Source: CAD feature listing. Evaluate the final solid. Frame: model axes, mm. A direction names the side the tool comes from. Give positions to 0.01 mm unless a question says otherwise; leave off trailing zeros. Order: outer loops, then holes, each group sorted by start corner. A loop starts at its lowest first (then second) coordinate and runs counter-clockwise, first axis right, second up. Notation, with made-up numbers: (-31.5, -11.75) - (-0.5, -11.75) arc R12 ccw to (-0.5, 2.25) - close; hole circle Ø2 at (57, 28). An arc over 180 degrees is marked (long way). Use CSV: the item, a comma, the result in double quotes.
```python
from build123d import *

# Parameters (mm, degrees)
SKETCH3_R               = 15.875
BOSS_EXTRUDE1_DEPTH     = 63.5
BOSS_EXTRUDE2_START     = -12.7
SKETCH4_W               = 63.5
SKETCH4_H               = 63.5
SKETCH4_R               = 15.875
SKETCH4_R_2             = 6.35
BOSS_EXTRUDE2_DEPTH     = 76.2
CUT_EXTRUDE1_REACH      = 147.497
CUT_EXTRUDE1_END_RADIUS = 6.35
SKETCH5_R               = 6.35


with BuildPart() as part:
    # Sketch3 → Boss-Extrude1 (new body)
    with BuildSketch(Plane(origin=(0, 0, 0), x_dir=(1, 0, 0), z_dir=(0, 1, 0))):
        with Locations(Location((0, 0, 0), (0, 0, 270))):
            Circle(SKETCH3_R)
    extrude(amount=BOSS_EXTRUDE1_DEPTH)


with BuildPart() as body_2:
    # Sketch4 → Boss-Extrude2 (new body)
    # profile 1 of 2: a face of its own
    with BuildSketch(Plane(origin=(0, 63.5, 0), x_dir=(1, 0, 0), z_dir=(0, 1, 0)).offset(BOSS_EXTRUDE2_START)):
        Rectangle(SKETCH4_W, SKETCH4_H)
        with Locations(Location((0, 0, 0), (0, 0, 270))):
            Circle(SKETCH4_R, mode=Mode.SUBTRACT)
    # profile 2 of 2: a face of its own
    with BuildSketch(Plane(origin=(0, 63.5, 0), x_dir=(1, 0, 0), z_dir=(0, 1, 0)).offset(BOSS_EXTRUDE2_START)):
        with Locations(Location((0, 0, 0), (0, 0, 270))):
            Circle(SKETCH4_R)
        with Locations(Location((0, 0, 0), (0, 0, 90))):
            Circle(SKETCH4_R_2, mode=Mode.SUBTRACT)
    extrude(amount=BOSS_EXTRUDE2_DEPTH)

    # Cut-Extrude1: up to this cylinder (the profile starts outside it)
    cut_extrude1_end = Plane(origin=(0, 95.25, 0), z_dir=(0, -1, 0)) * Cylinder(CUT_EXTRUDE1_END_RADIUS, 308.694, mode=Mode.PRIVATE)
    # Sketch5 → Cut-Extrude1 (cut, up to the surface)
    with BuildSketch(Plane.XY.offset(31.75), mode=Mode.PRIVATE) as cut_extrude1_sk1:
        with Locations((0, 95.25)):
            Circle(SKETCH5_R)
    cut_extrude1_tool1 = extrude(cut_extrude1_sk1.sketch, amount=-CUT_EXTRUDE1_REACH, mode=Mode.PRIVATE) - cut_extrude1_end
    add(cut_extrude1_tool1.solids().sort_by_distance((0, 95.25, 31.75))[0], mode=Mode.SUBTRACT)


with BuildPart() as part_1:
    add(part.part)

    # Combine1: union body 2
    add(body_2.part)


solid = part_1.part
```
Item 1: Section B-B on x = 0. Return the cut outline in (y, z) (3 decimals).
Filled in:
outline,"(0, -15.875) - (50.8, -15.875) - (50.8, -31.75) - (127, -31.75) - (127, -6.35) - (63.5, -6.35) - (63.5, 6.35) - (88.9, 6.35) - (88.9, 31.75) - (50.8, 31.75) - (50.8, 15.875) - (0, 15.875) - close; (101.6, 6.35) - (127, 6.35) - (127, 31.75) - (101.6, 31.75) - close"
Item 2: Mould query, pull axis X, two halves, no side actions, for faces 5 (the cylindrical face through (-1.907, 94.806, -6.057)), 6 (the flat face through (8, 127, 0)), 7 (the flat face through (-31.75, 88, 0)). Classes: released by +X, released by -X, zero draft, split by the parting line, or undercut.
Filled in:
face 5,"undercut"
face 6,"zero draft"
face 7,"released by -X"
Item 3: First-contact query: pin 1 (6 mm diameter, centred on x = 7.5, z = 19, fed in from -Y); pin 2 (1 mm diameter, centred on x = 4.5, y = 24.5, fed in from -Z); pin 3 (12 mm diameter, centred on x = -10.5, y = 22.5, fed in from +Z). Flat tips, straight axial feed; report the tip coordinate or a pass-through.
Filled in:
pin 1,"stops at y = 50.8"
pin 2,"stops at z = -15.36"
pin 3,"stops at z = 15.22"
Item 4: Section D-D on y = 95.25. Return the cut outline in (x, z).
Filled in:
outline,"(-31.75, -31.75) - (31.75, -31.75) - (31.75, 31.75) - (6.35, 31.75) - (6.35, 0) arc R6.35 cw to (-6.35, 0) - (-6.35, 31.75) - (-31.75, 31.75) - close"
Item 5: Section C-C on y = 74. Return the cut outline in (x, z).
Filled in:
outline,"(-31.75, -31.75) - (31.75, -31.75) - (31.75, 31.75) - (-31.75, 31.75) - close; hole circle Ø12.7 at (0, 0)"
Item 6: Set-up query: faces 1 (the cylindrical face through (-0.827, 101.546, 19.625)), 2 (the cylindrical face through (-15.497, 25.044, -3.441)), 3 (the flat face through (0, 88, 31.75)), 4 (the flat face through (0, 63.5, 0)). Return all of +Z, -Z, +X, -X, +Y, -Y with unobstructed straight access to the full face (end or side cutting, diameter ignored); none if empty.
Filled in:
face 1,"+Z"
face 2,"-Y"
face 3,"+Z, +X, -X, +Y, -Y"
face 4,"+Y"
Item 7: Section A-A on z = 20. Return the cut outline in (x, y).
Filled in:
outline,"(-31.75, 50.8) - (31.75, 50.8) - (31.75, 127) - (-31.75, 127) - close; hole circle Ø12.7 at (0, 95.25)"
Item 8: Material intervals for line 1 (X direction, y = 95.25, z = 9.5); line 2 (Y direction, x = 0, z = 13); line 3 (Y direction, x = -18, z = -18), sorted ascending. Write a range as from..to.
Filled in:
line 1,"x = -31.75..-6.35, 6.35..31.75"
line 2,"y = 0..88.9, 101.6..127"
line 3,"y = 50.8..127"
